Geometry check sheet. Reference: the model listing, model coordinates, mm. Face numbers are marked on the shaded views. A direction names the side the tool comes from. Round coordinates to 2 decimals unless told otherwise and drop trailing zeros. Loops run counter-clockwise (first coordinate to the right, second up) from the corner with the lowest first, then second, coordinate; pieces in that order, holes last. Notation, with made-up numbers: M 82.25,8.5 L 115.25,8.5 A25 cw 115.25,35.5 Z; hole C -1.75,19.5 d4. An arc over 180 degrees is marked long. Write item = value, one per line.
from build123d import *

# Parameters (mm, degrees)
SKETCH054_W             = 40
SKETCH054_H             = 60
PAD026_DEPTH            = 20
SKETCH055_W             = 76.736599
SKETCH055_H             = 75.902515
SKETCH055_W_2           = 30
SKETCH055_H_2           = 54
SKETCH055_W_3           = 6.212331
SKETCH055_H_3           = 3.975892
SKETCH055_W_4           = 5.404726
SKETCH055_H_4           = 4.286509
SKETCH055_W_5           = 10.809453
SKETCH055_H_5           = 4.472877
SKETCH055_W_6           = 5.031989
SKETCH055_H_6           = 11.120071
SKETCH055_W_7           = 5.094109
SKETCH055_H_7           = 10.188222
POCKET035_DEPTH         = 18
SKETCH056_W             = 9.119706
SKETCH056_H             = 14.092372
POCKET036_DEPTH         = 56.898491
POCKET036_FACE35_W      = 4.472877
POCKET036_FACE35_H      = 11.822582
POCKET037_DEPTH         = 31.511028
BODY012_PLACEMENT_ANGLE = 90


with BuildPart() as part:
    # Sketch054 → Pad026 (new body)
    with BuildSketch(Plane.XY):
        Rectangle(SKETCH054_W, SKETCH054_H)
    extrude(amount=PAD026_DEPTH)

    # Sketch055 (on Face6 of Pad026) → Pocket035 (cut)
    with BuildSketch(Plane.XY.offset(20)):
        with Locations((-3.081739, -0.215215)):
            Rectangle(SKETCH055_W, SKETCH055_H)
        with Locations((-5, 3)):
            Rectangle(SKETCH055_W_2, SKETCH055_H_2, mode=Mode.SUBTRACT)
        with Locations((-14.747609, -26.978939)):
            Rectangle(SKETCH055_W_3, SKETCH055_H_3, mode=Mode.SUBTRACT)
        with Locations((-4.901067, -27.009999)):
            Rectangle(SKETCH055_W_4, SKETCH055_H_4, mode=Mode.SUBTRACT)
        with Locations((8.300133, -27.041061)):
            Rectangle(SKETCH055_W_5, SKETCH055_H_5, mode=Mode.SUBTRACT)
        with Locations((14.981133, 21.337455)):
            Rectangle(SKETCH055_W_6, SKETCH055_H_6, mode=Mode.SUBTRACT)
        with Locations((15.012193, 8.136257)):
            Rectangle(SKETCH055_W_7, SKETCH055_H_7, mode=Mode.SUBTRACT)
    extrude(amount=-POCKET035_DEPTH, mode=Mode.SUBTRACT)

    # Sketch056 (on Face20 of Pocket035) → Pocket036 (cut, through all)
    with BuildSketch(Plane(origin=(0, 26.897491, 0), x_dir=(-1, 0, 0), z_dir=(0, 1, 0))):
        with Locations((-16.069881, 15.223603)):
            Rectangle(SKETCH056_W, SKETCH056_H)
    extrude(amount=-POCKET036_DEPTH, mode=Mode.SUBTRACT)

    # Pocket036 Face35 → Pocket037 (cut, through all)
    with BuildSketch(Plane(origin=(11.510028, -27.041061, 14.088709), x_dir=(0, -1, 0), z_dir=(1, 0, 0))):
        with Locations((1e-06, 0)):
            Rectangle(POCKET036_FACE35_W, POCKET036_FACE35_H)
    extrude(amount=-POCKET037_DEPTH, mode=Mode.SUBTRACT)


with BuildPart() as part_1:
    # Body012 placement: moved
    add(part.part.moved(Location((-27.6, 75, -1))).rotate(Axis((-27.6, 75, -1), (0, 1, 0)), BODY012_PLACEMENT_ANGLE))


solid = part_1.part
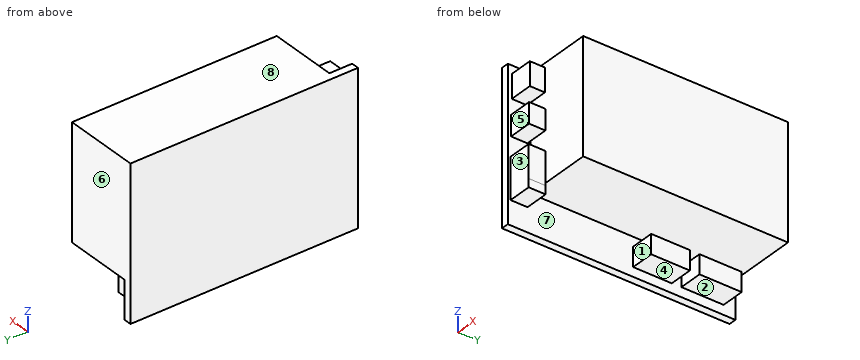
(1) Tool access check on the marked faces 1, 2, 3, 4 and 5. Record the directions out of +Z, -Z, +X, -X, +Y, -Y that give a thin tool (end or side, any length) a straight path to the whole face; none if there is none.
Result set:
face_1 = -Z, +X
face_2 = -Z, +X, +Y
face_3 = +Z, -Z, +X, -Y
face_4 = -Z, +X, +Y, -Y
face_5 = +Z, +X, -Y
(2) Sectioned sample at B-B on z = 11.5. Record the cut outline in (x, y).
Result set:
outline = M -27.6,45 L -25.6,45 L -25.6,46.03 L -19.42,46.03 L -19.42,50.01 L -25.6,50.01 L -25.6,51 L -7.6,51 L -7.6,105 L -27.6,105 Z
(3) Depth check by flat-ended pin: pin 1 Ø3 at (x, z) = (-10.5, 1) entering from -Y; pin 2 Ø5.5 at (y, z) = (96, -16.5) entering from +X; pin 3 Ø5.5 at (x, z) = (-22, -16.5) entering from +Y; pin 4 Ø1.5 at (x, z) = (-17.5, -15.5) entering from +Y. Enter the tip coordinate at first touch or a pass-through.
Result set:
pin_1 = 51
pin_2 = -19.42
pin_3 = 101.9
pin_4 = through
(4) Release check for a two-part mould opening along Z. For the marked faces 6, 7 and 8 record: released by +Z, released by -Z, zero draft, split by the parting line, or undercut.
Result set:
face_6 = zero draft
face_7 = undercut
face_8 = released by +Z
(5) Material ranges on line 1 along Y through (x, z) = (-20.75, 3.5); line 2 along Y through (x, z) = (-21.5, 14.5); line 3 along Y through (x, z) = (-13, 15.5), recorded low to high. Write a range as from..to.
Result set:
line_1 = 45.85..50.13, 51..105
line_2 = 46.03..50.01, 51..105
line_3 = 51..105
(6) Sectioned sample at D-D on z = 6. Record the cut outline in (x, y), then the cut area to 3 significant figures.
Result set:
outline = M -27.6,45 L -25.6,45 L -25.6,45.85 L -19.42,45.85 L -19.42,50.13 L -25.6,50.13 L -25.6,51 L -7.6,51 L -7.6,105 L -27.6,105 Z
area = 1,120 mm2
(7) Sectioned sample at C-C on y = 62. Record the cut outline in (x, z).
Result set:
outline = M -27.6,-21 L -25.6,-21 L -25.6,-11 L -7.6,-11 L -7.6,19 L -27.6,19 Z
(8) Sectioned sample at A-A on x = -21.75. Record the cut outline in (y, z), then the cut area to 3 significant figures.
Result set:
outline = M 45.72,-14.7 L 50.2,-14.7 L 50.2,-3.9 L 45.72,-3.9 Z; M 45.85,1.2 L 50.13,1.2 L 50.13,6.6 L 45.85,6.6 Z; M 46.03,10.64 L 50.01,10.64 L 50.01,16.85 L 46.03,16.85 Z; M 51,-11 L 105,-11 L 105,19 L 51,19 Z; M 78.04,-18.56 L 88.23,-18.56 L 88.23,-13.47 L 78.04,-13.47 Z; M 90.78,-18.5 L 101.9,-18.5 L 101.9,-13.47 L 90.78,-13.47 Z
area = 1,820 mm2
